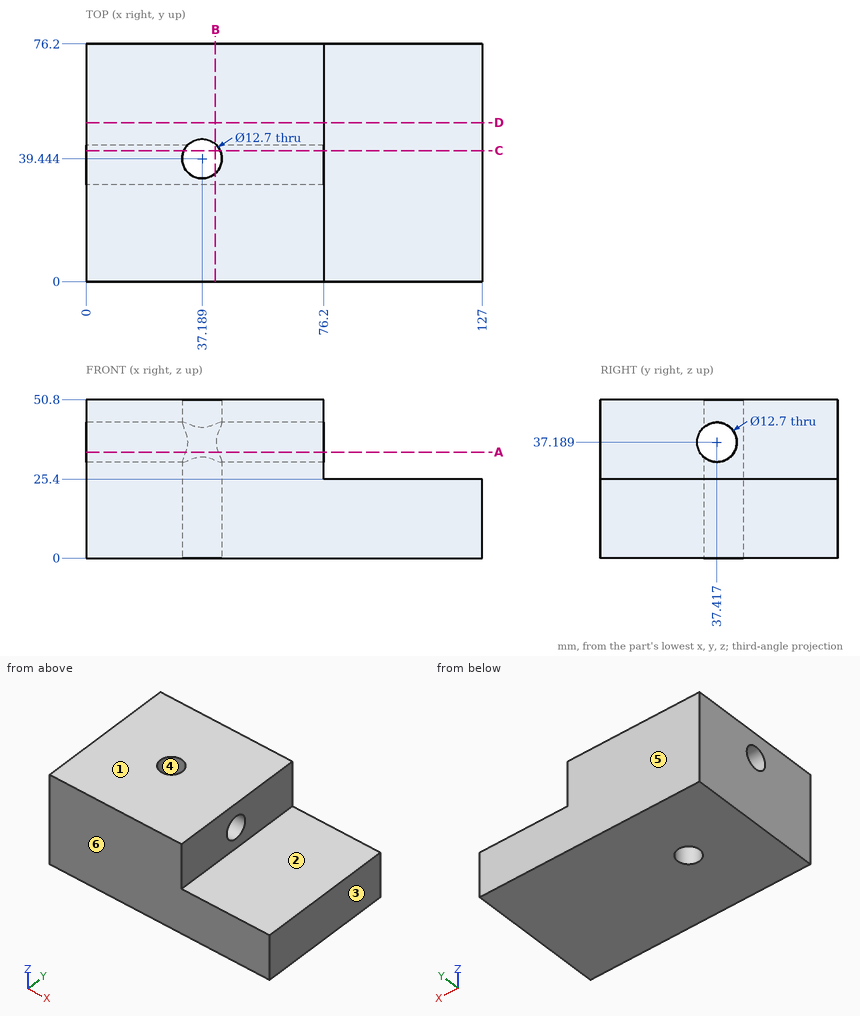
Design review of the part shown in the three views and the two pictorial views. Dimensions are in mm from the part's minimum x, y and z. A direction names the side the tool comes from. Coordinates: 2 decimals unless noted, no trailing zeros. Order: outer loops, then holes, each group sorted by start corner. A loop starts at its lowest first (then second) coordinate and runs counter-clockwise, first axis right, second up.
1) For the marked faces 1 and 2, list the 3-axis set-ups (+Z, -Z, +X, -X, +Y, -Y) from which the entire face can be reached by the end or side of a thin tool; tool diameter is ignored.
2) Mouldability with a two-part tool opening along Y and no side actions: class the marked faces 3, 4, 5 and 6 as +Y half, -Y half, draft (parallel to the pull), parting line (faces both ways), or undercut.
3) Wall thickness on line 1 along X through (y, z) = (19, 37.5); line 2 along Z through (x, y) = (103.5, 52); line 3 along Z through (x, y) = (28, 36): over which ranges is each line inside the solid? List them lowest first.
4) Clearance check with a flat-ended pin moving along its axis: pin 1 (20.5 mm diameter, centred on y = 55.5, z = 43.5, fed in from +X). State where the tip first meets the part, or that it passes through.
5) Take a section at D-D, the plane y = 51. Give the boundary of the cut face in (x, z).
6) Take a section at C-C, the plane y = 42. Give the boundary of the cut face in (x, z) (1 decimal).
7) Take a section at A-A, the plane z = 34. Give the boundary of the cut face in (x, y), and give its area (3 significant figures).
8) Take a section at B-B, the plane x = 41.5. Give the boundary of the cut face in (y, z), and give its area (3 significant figures).
Returned:
1. face 1: +Z, +X, -X, +Y, -Y
1. face 2: +Z, +X, +Y, -Y
2. face 3: draft
2. face 4: undercut
2. face 5: +Y half
2. face 6: -Y half
3. line 1: x = 0 to 76.2
3. line 2: z = 0 to 25.4
3. line 3: z = 0 to 31, 43.38 to 50.8
4. pin 1: stops at x = 76.2
5. outline: (0, 0) - (127, 0) - (127, 25.4) - (76.2, 25.4) - (76.2, 50.8) - (0, 50.8) - close
6. outline: (0, 0) - (31.4, 0) - (31.4, 32.8) - (0, 32.8) - close; (0, 41.6) - (31.4, 41.6) - (31.4, 50.8) - (0, 50.8) - close; (43, 0) - (127, 0) - (127, 25.4) - (76.2, 25.4) - (76.2, 32.8) - (43, 32.8) - close; (43, 41.6) - (76.2, 41.6) - (76.2, 50.8) - (43, 50.8) - close
7. outline: (0, 0) - (76.2, 0) - (76.2, 31.93) - (0, 31.93) - close; (0, 42.91) - (31.87, 42.91) arc R6.35 cw to (42.51, 42.91) - (76.2, 42.91) - (76.2, 76.2) - (0, 76.2) - close
7. area: 4,950 mm2
8. outline: (0, 0) - (34.78, 0) - (34.78, 31.41) arc R6.35 cw to (34.78, 42.97) - (34.78, 50.8) - (0, 50.8) - close; (44.11, 0) - (76.2, 0) - (76.2, 50.8) - (44.11, 50.8) - close
8. area: 3,370 mm2
